Here's the drawing with two shaded views (mm, measured from the low corner). I have some questions. Give positions to 0.01 mm unless a question says otherwise; leave off trailing zeros. Loops run counter-clockwise (first coordinate to the right, second up) from the corner with the lowest first, then second, coordinate; pieces in that order, holes last. Notation, with made-up numbers: M 20.5,37 L 69.5,37 A11 ccw 69.5,49 Z; hole C 68.5,-37.5 d9. An arc over 180 degrees is marked long. Put each result on its own line as item: value. Start each with the question number.
1) Imagine slicing it at B-B (x = 2.9). Write out the boundary of the cut face in (y, z), then the cut area to 3 significant figures.
2) Imagine slicing it at C-C (y = 2). Write out the boundary of the cut face in (x, z), then the cut area to 3 significant figures.
3) Imagine slicing it at A-A (z = 4.75). Write out the boundary of the cut face in (x, y), then the cut area to 3 significant figures.
4) If we mould it in two halves opening along Y, with no side actions, what happens to the marked faces 1, 2 and 3? For each: +Y half, -Y half, draft (parallel to the pull), parting line (faces both ways), or undercut.
5) Please list where these lines run through material, in increasing order: line 1 along Y through (x, z) = (3, 8.45); line 2 along Y through (x, z) = (3, 3.7); line 3 along X through (y, z) = (2, 4.15). Write a range as from..to.
6) Imagine slicing it at D-D (z = 9.75). Write out the boundary of the cut face in (x, y), then the cut area to 3 significant figures.
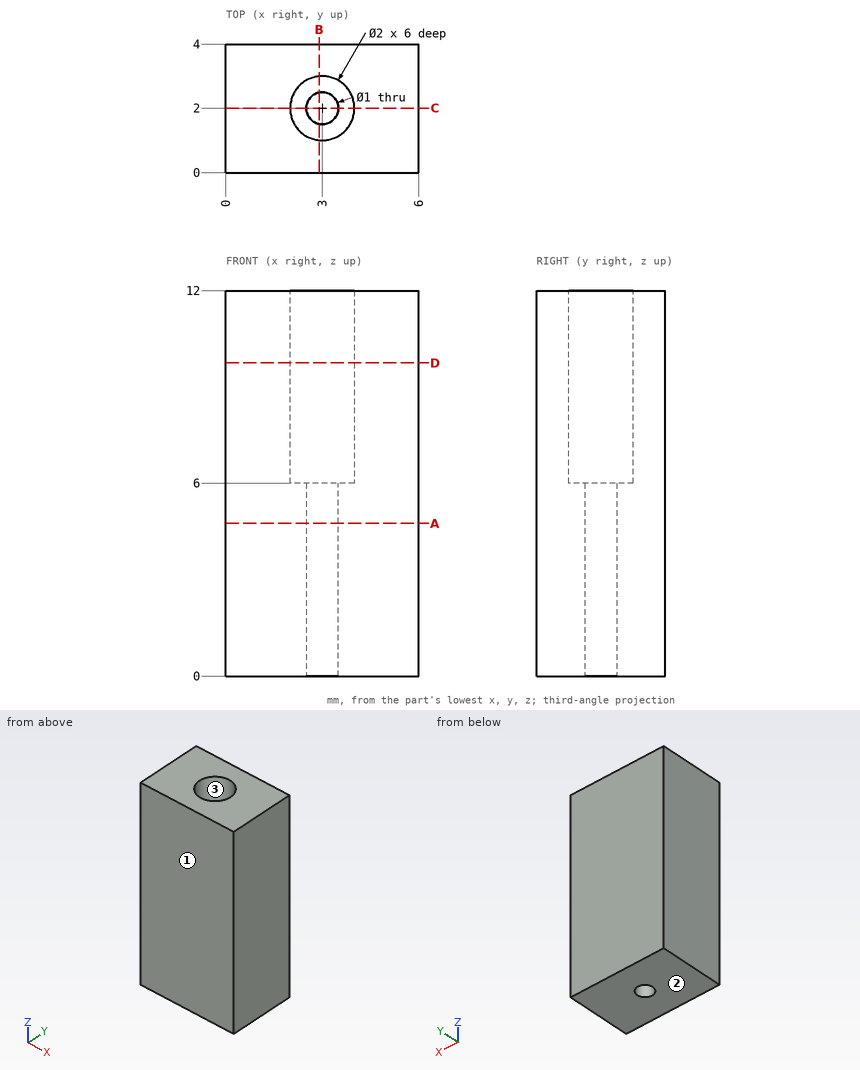
Recorded:
1. outline: M 0,0 L 1.51,0 L 1.51,6 L 1.01,6 L 1.01,12 L 0,12 Z; M 2.49,0 L 4,0 L 4,12 L 2.99,12 L 2.99,6 L 2.49,6 Z
1. area: 30.2 mm²
2. outline: M 0,0 L 2.5,0 L 2.5,6 L 2,6 L 2,12 L 0,12 Z; M 3.5,0 L 6,0 L 6,12 L 4,12 L 4,6 L 3.5,6 Z
2. area: 54.0 mm²
3. outline: M 0,0 L 6,0 L 6,4 L 0,4 Z; hole C 3,2 d1
3. area: 23.2 mm²
4. face 1: -Y half
4. face 2: draft
4. face 3: undercut
5. line 1: 0..1, 3..4
5. line 2: 0..1.5, 2.5..4
5. line 3: 0..2.5, 3.5..6
6. outline: M 0,0 L 6,0 L 6,4 L 0,4 Z; hole C 3,2 d2
6. area: 20.9 mm²
